Can you work these out from the model? Positions are in its coordinate system, mm. Give positions to 0.01 mm unless a question says otherwise; leave off trailing zeros. Loops run counter-clockwise (first coordinate to the right, second up) from the corner with the lowest first, then second, coordinate; pieces in that order, holes last. Notation, with made-up numbers: (81.25, 14.25) - (94.25, 14.25) arc R25 ccw to (94.25, 50.25) - close; hole circle Ø8 at (58.25, -26.75). An arc over 180 degrees is marked (long way). Answer in a Markdown table with one row per item.
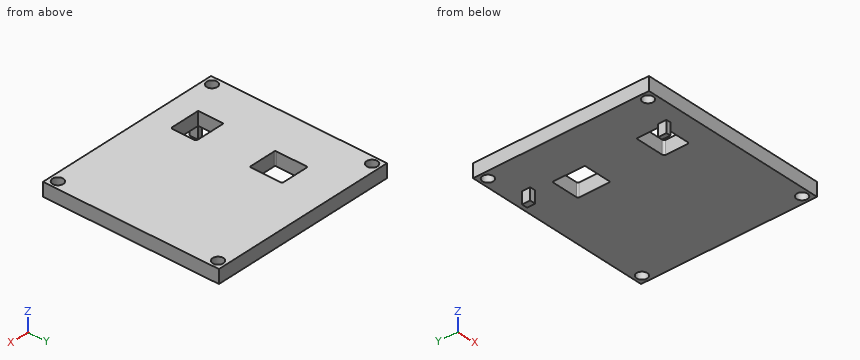
from build123d import *

# Parameters (mm, degrees)
SKIZZE1_R                       = 2
AUFSATZ_LINEAR_AUSTRAGEN1_DEPTH = 5
SKIZZE2_W                       = 1.65
SKIZZE2_H                       = 4.42
AUFSATZ_LINEAR_AUSTRAGEN2_DEPTH = 3
SKIZZE3_W                       = 2.08
SKIZZE3_H                       = 4.42
AUFSATZ_LINEAR_AUSTRAGEN3_DEPTH = 3


with BuildPart() as part:
    # Skizze1 → Aufsatz-Linear austragen1 (new body)
    # profile 1 of 2: a face of its own
    with BuildSketch(Plane.XY):
        Polygon((70, 5.85), (70, 59.15), (13.85, 59.15), (13.85, 58.15), (10.85, 58.15), (10.85, 59.15), (5.85, 59.15), (5.85, 5.85), (10.85, 5.85), (10.85, 6.85), (13.85, 6.85), (13.85, 5.85), align=None)
        with BuildLine():
            Line((26.7, 17.485), (26.7, 9.485))
            ThreePointArc((26.7, 9.485), (26.494974747, 8.990025253), (26, 8.785))
            Line((26, 8.785), (15.3, 8.785))
            Line((15.3, 8.785), (15.3, 18.185))
            Line((15.3, 18.185), (26, 18.185))
            ThreePointArc((26, 18.185), (26.494974747, 17.979974747), (26.7, 17.485))
        make_face(mode=Mode.SUBTRACT)
        with BuildLine():
            Line((16.34, 49.85), (25.99, 49.85))
            Line((25.99, 49.85), (26.09, 49.85))
            ThreePointArc((26.09, 49.85), (26.415269119, 49.715269119), (26.55, 49.39))
            Line((26.55, 49.39), (26.55, 38.27))
            ThreePointArc((26.55, 38.27), (26.415269119, 37.944730881), (26.09, 37.81))
            Line((26.09, 37.81), (25.99, 37.81))
            Line((25.99, 37.81), (16.34, 37.81))
            ThreePointArc((16.34, 37.81), (16.05008622, 37.93008622), (15.93, 38.22))
            Line((15.93, 38.22), (15.93, 49.44))
            ThreePointArc((15.93, 49.44), (16.05008622, 49.72991378), (16.34, 49.85))
        make_face(mode=Mode.SUBTRACT)
    # profile 2 of 2: a face of its own
    with BuildSketch(Plane.XY):
        Polygon((13.85, 59.15), (70, 59.15), (70, 65), (0, 65), (0, 0), (70, 0), (70, 5.85), (13.85, 5.85), (13.85, 6.85), (10.85, 6.85), (10.85, 5.85), (5.85, 5.85), (5.85, 59.15), (10.85, 59.15), (10.85, 58.15), (13.85, 58.15), align=None)
        with Locations((2.925, 2.925)):
            Circle(SKIZZE1_R, mode=Mode.SUBTRACT)
        with Locations((67.075, 2.925)):
            Circle(SKIZZE1_R, mode=Mode.SUBTRACT)
        with Locations((2.925, 62.075)):
            Circle(SKIZZE1_R, mode=Mode.SUBTRACT)
        with Locations((67.075, 62.075)):
            Circle(SKIZZE1_R, mode=Mode.SUBTRACT)
    extrude(amount=AUFSATZ_LINEAR_AUSTRAGEN1_DEPTH)

    # Skizze2 → Aufsatz-Linear austragen2 (add)
    with BuildSketch(Plane(origin=(0, 5.85, 0), x_dir=(1, 0, 0), z_dir=(0, 1, 0))):
        with Locations((14.675, 2.21)):
            Rectangle(SKIZZE2_W, SKIZZE2_H)
    extrude(amount=AUFSATZ_LINEAR_AUSTRAGEN2_DEPTH)

    # Skizze3 → Aufsatz-Linear austragen3 (add)
    with BuildSketch(Plane.XZ.offset(-59.15)):
        with Locations((14.89, -2.21)):
            Rectangle(SKIZZE3_W, SKIZZE3_H)
    extrude(amount=AUFSATZ_LINEAR_AUSTRAGEN3_DEPTH)


solid = part.part
Q1. Imagine slicing it at A-A, the plane y = 46.5. Write out the boundary of the cut face in (x, z), and give its area (3 significant figures).
Checked values:
| item | result |
|---|---|
| outline | (0, 0) - (15.93, 0) - (15.93, 5) - (0, 5) - close; (26.55, 0) - (70, 0) - (70, 5) - (26.55, 5) - close |
| area | 297 mm² |
Q2. For pin 1 (12 mm diameter, centred on x = 33.5, y = 22, fed in from -Z); pin 2 (0.5 mm diameter, centred on x = 14.5, z = -3.5, fed in from -Y); pin 3 (1.3 mm diameter, centred on x = 14.5, z = -1.5, fed in from +Y), each with a flat end and sliding along its axis, tell me the tip position at first contact or that it passes through.
Checked values:
| item | result |
|---|---|
| pin 1 | stops at z = 0 |
| pin 2 | stops at y = 5.85 |
| pin 3 | stops at y = 59.15 |
Q3. Imagine slicing it at B-B, the plane x = 18.5. Write out the boundary of the cut face in (y, z) (3 decimals), and give its area (3 significant figures).
Checked values:
| item | result |
|---|---|
| outline | (0, 0) - (8.785, 0) - (8.785, 5) - (0, 5) - close; (18.185, 0) - (37.81, 0) - (37.81, 5) - (18.185, 5) - close; (49.85, 0) - (65, 0) - (65, 5) - (49.85, 5) - close |
| area | 218 mm² |
Q4. If I drill on line 1 (X direction, y = 45.5, z = 1); line 2 (X direction, y = 16.5, z = 2.75); line 3 (Z direction, x = 36, y = 32), over which ranges is the centre line in solid material (lowest first)? Write a range as [from, to].
Checked values:
| item | result |
|---|---|
| line 1 | x = [0, 15.93], [26.55, 70] |
| line 2 | x = [0, 15.3], [26.7, 70] |
| line 3 | z = [0, 5] |
Q5. Imagine slicing it at C-C, the plane z = -2.5. Write out the boundary of the cut face in (x, y), and give its area (3 significant figures).
Checked values:
| item | result |
|---|---|
| outline | (13.85, 5.85) - (15.5, 5.85) - (15.5, 8.85) - (13.85, 8.85) - close; (13.85, 56.15) - (15.93, 56.15) - (15.93, 59.15) - (13.85, 59.15) - close |
| area | 11.2 mm² |
Q6. Imagine slicing it at D-D, the plane z = 1.5. Write out the boundary of the cut face in (x, y) (3 decimals).
Checked values:
| item | result |
|---|---|
| outline | (0, 0) - (70, 0) - (70, 65) - (0, 65) - close; hole circle Ø4 at (2.925, 2.925); hole circle Ø4 at (2.925, 62.075); hole (15.3, 8.785) - (26, 8.785) arc R0.7 ccw to (26.7, 9.485) - (26.7, 17.485) arc R0.7 ccw to (26, 18.185) - (15.3, 18.185) - close; hole (15.93, 38.22) arc R0.41 ccw to (16.34, 37.81) - (26.09, 37.81) arc R0.46 ccw to (26.55, 38.27) - (26.55, 49.39) arc R0.46 ccw to (26.09, 49.85) - (16.34, 49.85) arc R0.41 ccw to (15.93, 49.44) - close; hole circle Ø4 at (67.075, 2.925); hole circle Ø4 at (67.075, 62.075) |
